For this review, take the finished solid that the model builds, in its own axes (mm). Coordinates: 2 decimals unless noted, no trailing zeros. Order: outer loops, then holes, each group sorted by start corner. A loop starts at its lowest first (then second) coordinate and runs counter-clockwise, first axis right, second up. Notation, with made-up numbers: (-31.5, 14.25) -> (4.5, 14.25) arc R21 cw to (4.5, 22.25) -> close; hole circle Ø7 at (-27, 52). An arc over 180 degrees is marked (long way). Write item = value, one per line. Start each with the question number.
1) Wall thickness on probe 1 along Z at (x, y) = (253.5, -17); probe 2 along X at (y, z) = (-25, 150); probe 3 along X at (y, z) = (19, 162): over which ranges is each line inside the solid? List them lowest first. Write a range as [from, to].
2) Consider section A-A on y = -14. Give the boundary of the cut face in (x, z), and give its area (3 significant figures).
3) Insertion check: pin 1 Ø3 at (x, y) = (219, 13) entering from +Z; pin 2 Ø1.5 at (y, z) = (-12, 83) entering from +X. Each pin has a flat end and moves straight along its axis. Give the tip position at first contact, or say it passes through.
from build123d import *

# Parameters (mm, degrees)
F1_DEPTH = 34.925
F2_R     = 5.08


with BuildPart() as f1:
    # F0 (on Front) → F1 (new body, symmetric)
    with BuildSketch(Plane.XZ):
        Polygon((0, 177.8), (0, 0), (304.8, 0), (304.8, 53.975), (76.2, 177.8), align=None)
    extrude(amount=F1_DEPTH, both=True)

    # F2
    f2_edges = [f1.edges().sort_by_distance(p)[0] for p in [
        (38.1, -34.925, 177.8),
        (0, -34.925, 88.9),
        (152.4, -34.925, 0),
        (304.8, -34.925, 26.9875),
        (190.5, -34.925, 115.8875),
        (38.1, 34.925, 177.8),
        (0, 34.925, 88.9),
        (152.4, 34.925, 0),
        (304.8, 34.925, 26.9875),
        (190.5, 34.925, 115.8875),
        (0, 0, 177.8),
        (76.2, 0, 177.8),
        (304.8, 0, 53.975),
        (0, 0, 0),
        (304.8, 0, 0),
    ]]
    fillet(f2_edges, radius=F2_R)


solid = f1.part
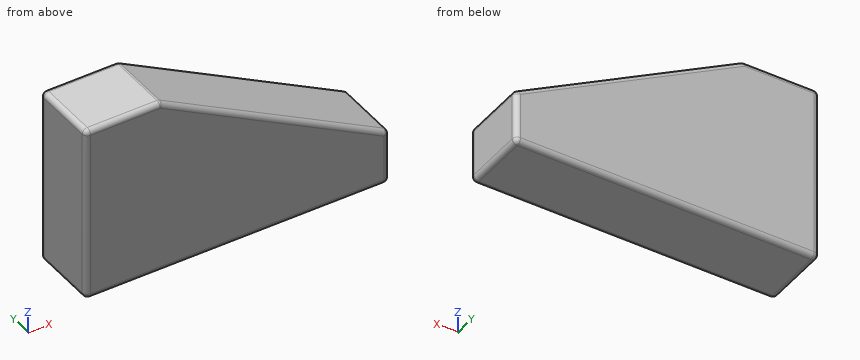
Answer sheet:
q1.probe_1 = [0, 81.76]
q1.probe_2 = [0, 127.52]
q1.probe_3 = [0, 105.37]
q2.outline = (0, 5.08) arc R5.08 ccw to (5.08, 0) -> (299.72, 0) arc R5.08 ccw to (304.8, 5.08) -> (304.8, 50.95) arc R5.08 ccw to (302.14, 55.42) -> (77.33, 177.19) arc R5.08 ccw to (74.91, 177.8) -> (5.08, 177.8) arc R5.08 ccw to (0, 172.72) -> close
q2.area = 40,000 mm2
q3.pin_1 = 101.26
q3.pin_2 = 252.6
